For this review, take the finished solid that the model builds, in its own axes (mm). A direction names the side the tool comes from. Round coordinates to 2 decimals unless told otherwise and drop trailing zeros. Order: outer loops, then holes, each group sorted by start corner. A loop starts at its lowest first (then second) coordinate and runs counter-clockwise, first axis right, second up.
Solid Edge part; units mm, degrees
sketch "Sketch1" plane through (0, 0, 0) normal (0, 0, 1) x (1, 0, 0)
  line L0 (62.2876, -20.4159) -> (62.2876, -4.3754)
  arc A0 (52.7547, 6.7636) -> (62.2876, -4.3754) centre (51.0132, -4.3754) cw
  arc A1 (40.1391, 9.8624) -> (52.7547, 6.7636) centre (64.4659, 81.6715) ccw
  arc A2 (25.0937, 1.0714) -> (30.5929, -13.6417) centre (35.281, -3.5053) ccw
  line L1 (30.5929, -13.6417) -> (33.6031, -15.0339)
  arc A3 (33.6031, -15.0339) -> (35.1927, -15.5836) centre (37.1297, -7.4088) ccw
  arc A4 (35.1927, -15.5836) -> (35.4622, -17.051) centre (35.0049, -16.3765) cw
  line L2 (35.4622, -17.051) -> (34.4237, -17.755)
  arc A5 (34.4237, -17.755) -> (29.3666, -18.4657) centre (31.171, -12.9576) cw
  line L3 (29.3666, -18.4657) -> (28.4941, -18.1799)
  arc A6 (20.5329, 3.1204) -> (28.4941, -18.1799) centre (35.281, -3.5053) ccw
  arc A7 (20.5329, 3.1204) -> (41.2336, 14.7729) centre (38.7764, -5.0756) cw
  arc A8 (41.2336, 14.7729) -> (56.3598, 11.3191) centre (64.4659, 81.6715) ccw
  arc A9 (56.3598, 11.3191) -> (62.2876, 16.6032) centre (56.9686, 16.6032) ccw
  line L4 (62.2876, 16.6032) -> (62.2876, 23.8866)
  line L5 (62.2876, 23.8866) -> (67.2703, 23.8866)
  line L6 (67.2703, 23.8866) -> (67.2703, -20.4159)
  line L7 (62.2876, -20.4159) -> (67.2703, -20.4159)
  arc A10 (25.0938, 1.0714) -> (40.1391, 9.8624) centre (38.7764, -5.0756) cw
extrude "Protrusion1" add sketch "Sketch1" along normal blind 15
sketch "Sketch2" plane through (62.2876, -7.2627, 12.5) normal (-1, 0, 0) x (0, -1, 0)
  circle A0 centre (0, -5) radius 2
extrude "ScavoEstrusione_1" cut sketch "Sketch2" along normal mid plane 363.09
sketch "Sketch3" plane through (62.2876, -7.2627, 12.5) normal (-1, 0, 0) x (0, -1, 0)
  circle A0 centre (0, -5) radius 3
extrude "ScavoEstrusione_2" cut sketch "Sketch3" along normal blind 211.9198
fillet "Rotondo_1" radius 3 1 edges at (62.2876, -7.2627, 5.5)
fillet "Rotondo_3" radius 13 1 edges at (40.1391, 9.8624, 7.5)
fillet "Rotondo_4" radius 19 1 edges at (41.2336, 14.7729, 7.5)
Q1. Tool access review of faces 4 (the face through (50.102, 12.326, 7.395)), 5 (the face through (24.863, -7.529, 4.062)), 6 (the face through (62.288, 20, 7)), 7 (the face through (22.811, -10.124, 6.599)), 8 (the face through (59.506, 3.04, 7.395)): name each direction out of +Z, -Z, +X, -X, +Y, -Y from which nothing blocks a thin tool from reaching the whole face with its end or side.
Q2. Clearance check with flat-ended pins moving along their axes: pin 1 (8 mm diameter, centred on x = 47.5, z = 4.5, fed in from +Y); pin 2 (6 mm diameter, centred on x = 38.5, z = 8, fed in from +Y); pin 3 (6 mm diameter, centred on x = 46, z = 11.5, fed in from +Y). State where each tip first meets the part, or that it passes through.
Q3. Take a section at A-A, the plane y = 20.5. State the section outline as (x, z) points.
Q4. Wall thickness on line 1 (Y direction, x = 66, z = 7.5); line 2 (X direction, y = -4, z = 2.25); line 3 (X direction, y = -16, z = 13.25): over which ranges is each line inside the solid? List them lowest first.
Q5. Mouldability with a two-part tool opening along X and no side actions: class faces 1 (the face through (67.27, 2, 7)), 2 (the face through (34.395, -15.352, 7.395)), 3 (the face through (65, -20.416, 7)) as +X half, -X half, draft (parallel to the pull), parting line (faces both ways), or undercut.
Q6. Take a section at B-B, the plane x = 59. State the section outline as (y, z) points.
Working result:
1. face 4: +Z, -Z, +Y
1. face 5: +Z, -Z
1. face 6: +Z, -Z, -X, +Y
1. face 7: -X
1. face 8: +Z, -Z, -Y
2. pin 1: stops at y = 14.03
2. pin 2: stops at y = 14.77
2. pin 3: stops at y = 14.16
3. outline: (62.29, 0) - (67.27, 0) - (67.27, 15) - (62.29, 15) - close
4. line 1: y = -20.42 to -9.26, -5.26 to 23.89
4. line 2: x = 19.12 to 24.12, 62.28 to 67.27
4. line 3: x = 25.02 to 35.73, 62.29 to 67.27
5. face 1: +X half
5. face 2: undercut
5. face 3: draft
6. outline: (3.58, 0) - (11.69, 0) - (11.69, 15) - (3.58, 15) - close
